Work out the finished part from the listing and answer in its coordinate system (mm). A direction names the side the tool comes from. Round coordinates to 2 decimals unless told otherwise and drop trailing zeros. Loops run counter-clockwise (first coordinate to the right, second up) from the corner with the lowest first, then second, coordinate; pieces in that order, holes last.
Autodesk Inventor part; units mm, degrees
ref_plane "YZ Plane" through (0, 0, 0) normal (1, 0, 0) x (0, 1, 0)
ref_plane "XZ Plane" through (0, 0, 0) normal (0, 1, 0) x (-1, 0, 0)
ref_plane "XY Plane" through (0, 0, 0) normal (0, 0, 1) x (1, 0, 0)
sketch "Sketch1" plane through (0, 0, 0) normal (0, 0, 1) x (1, 0, 0)
  circle A0 centre (0, 0) radius 53.9125
  circle A1 centre (0, 0) radius 61.9125
  line L0 (-3.6662, 6.35) -> (3.6662, 6.35)
  line L1 (3.6662, 6.35) -> (7.3323, 0)
  line L2 (7.3323, 0) -> (3.6662, -6.35)
  line L3 (3.6662, -6.35) -> (-3.6662, -6.35)
  line L4 (-3.6662, -6.35) -> (-7.3323, 0)
  line L5 (-7.3323, 0) -> (-3.6662, 6.35)
  circle A2 centre (0, 0) radius 48.9125
  circle A3 centre (0, 0) radius 15.5
  point P0 (0, -6.35)
  dimension "d0" = 8
  dimension "d2" = 12.7
  dimension "d7" = 123.825
  dimension "d8" = 13
  dimension "d13" = 31
extrude "Extrusion1" add sketch "Sketch1" along normal mid plane 12.7 contours A0 | A1 | A2 | A3
extrude "Extrusion2" add sketch "Sketch1" along normal mid plane 20.32 contours A1
extrude "Extrusion3" add sketch "Sketch1" along normal blind 10 contours A0
extrude "Extrusion4" add sketch "Sketch1" against normal blind 10 contours A0
extrude "Extrusion5" add sketch "Sketch1" along normal mid plane 15.24 contours A3
properties part number "hjul"
1. Determine the mould class of faces 4 (the face through (-13.42, -60.44, 0.14)), 5 (the face through (5.525, -3.131, -0.107)), 6 (the face through (-2.018, 15.368, -6.976)), 7 (the face through (-19, 51, 10.16)) for opening direction X: +X half, -X half, draft (parallel to the pull), parting line (faces both ways), or undercut.
Answer key:
face 4: parting line
face 5: undercut
face 6: undercut
face 7: draft
2. Which of the six approach directions +Z, -Z, +X, -X, +Y, -Y give full straight-line access (tool end or side, diameter ignored) to faces 1 (the face through (-2.018, -15.368, 6.976)), 2 (the face through (12, -48, -10)), 3 (the face through (0, -6.35, 0))?
Answer key:
face 1: +Z
face 2: -Z
face 3: +Z, -Z
3. Consider probe 1 along Y at (x, z) = (-1, -3); probe 2 along Y at (x, z) = (0, -8.15); probe 3 along Z at (x, y) = (22, -23). Determine where each line is inside the solid, lowest interval first.
Answer key:
probe 1: y = -61.9 to -6.35, 6.35 to 61.9
probe 2: y = -61.91 to -48.91, 48.91 to 61.91
probe 3: z = -6.35 to 6.35
4. Given pin 1 (4 mm diameter, centred on x = 15.5, z = 6.5, fed in from +Y); pin 2 (2 mm diameter, centred on x = 1, z = -2.5, fed in from +Y); pin 3 (2 mm diameter, centred on x = -0.5, z = 3.5, fed in from -Y), each flat-ended and moving along its own axis, determine where each tip first touches the part or whether it passes through.
Answer key:
pin 1: stops at y = 60.42
pin 2: stops at y = 61.91
pin 3: stops at y = -61.91
5. Find section D-D (x = -45.5). Write down the section's boundary in (y, z), then the cut area to 3 significant figures.
Answer key:
outline: (-41.99, -10.16) - (-28.92, -10.16) - (-28.92, -10) - (-17.95, -10) - (-17.95, -6.35) - (17.95, -6.35) - (17.95, -10) - (28.92, -10) - (28.92, -10.16) - (41.99, -10.16) - (41.99, 10.16) - (28.92, 10.16) - (28.92, 10) - (17.95, 10) - (17.95, 6.35) - (-17.95, 6.35) - (-17.95, 10) - (-28.92, 10) - (-28.92, 10.16) - (-41.99, 10.16) - close
area: 1,430 mm2
6. Find section C-C (y = 44). Write down the section's boundary in (x, z).
Answer key:
outline: (-43.56, -10.16) - (-31.15, -10.16) - (-31.15, -10) - (-21.36, -10) - (-21.36, -6.35) - (21.36, -6.35) - (21.36, -10) - (31.15, -10) - (31.15, -10.16) - (43.56, -10.16) - (43.56, 10.16) - (31.15, 10.16) - (31.15, 10) - (21.36, 10) - (21.36, 6.35) - (-21.36, 6.35) - (-21.36, 10) - (-31.15, 10) - (-31.15, 10.16) - (-43.56, 10.16) - close
